Could you check a few things on this drawing? It's one solid part, dimensions in mm from its lowest x, y, z. Round coordinates to 2 decimals unless told otherwise and drop trailing zeros. Loops run counter-clockwise (first coordinate to the right, second up) from the corner with the lowest first, then second, coordinate; pieces in that order, holes last. Notation, with made-up numbers: (-29, -22) -> (-10, -22) arc R21 ccw to (-10, 15) -> close; hole circle Ø9 at (66, -9.5). An arc over 180 degrees is marked (long way). Write each question's results on one line, items separated by ' | '.
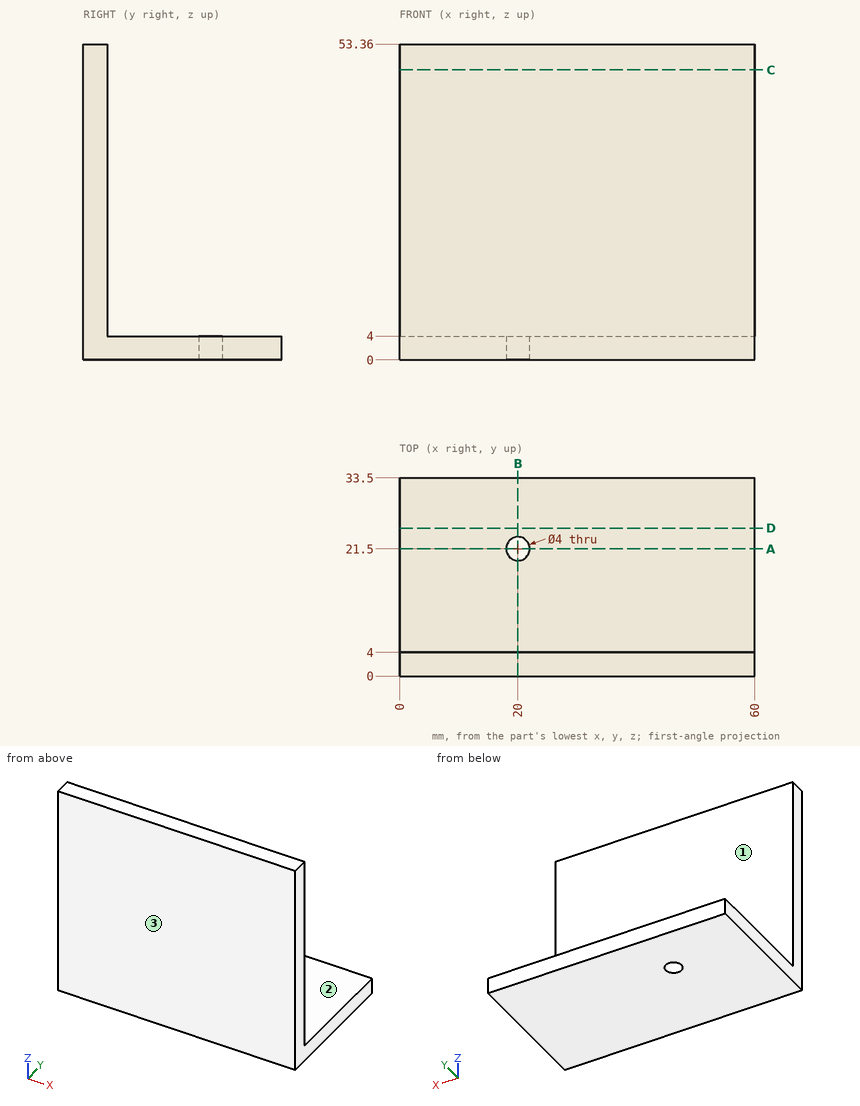
1) I need wall thicknesses on line 1 (Z direction, x = 25.5, y = 30.5); line 2 (Y direction, x = 20, z = 1). Which ranges of each line are inside material? Lowest first, please.
Model answer:
line 1: z = 0 to 4 | line 2: y = 0 to 19.5, 23.5 to 33.5
2) I want a section at B-B, the plane x = 20. Write out the boundary of the cut face in (y, z), plus the area to 3 significant figures.
Model answer:
outline: (0, 0) -> (19.5, 0) -> (19.5, 4) -> (4, 4) -> (4, 53.36) -> (0, 53.36) -> close; (23.5, 0) -> (33.5, 0) -> (33.5, 4) -> (23.5, 4) -> close | area: 315 mm2
3) I want a section at C-C, the plane z = 49. Write out the boundary of the cut face in (x, y).
Model answer:
outline: (0, 0) -> (60, 0) -> (60, 4) -> (0, 4) -> close
4) I want a section at A-A, the plane y = 21.5. Write out the boundary of the cut face in (x, z).
Model answer:
outline: (0, 0) -> (18, 0) -> (18, 4) -> (0, 4) -> close; (22, 0) -> (60, 0) -> (60, 4) -> (22, 4) -> close
5) If we mould it in two halves opening along Y, with no side actions, what happens to the marked faces 1, 2 and 3? For each: released by +Y, released by -Y, zero draft, split by the parting line, or undercut.
Model answer:
face 1: released by +Y | face 2: zero draft | face 3: released by -Y
6) I'm going to push flat-ended pins straight in: pin 1 (15 mm diameter, centred on x = 23.5, z = 36.5, fed in from +Y); pin 2 (3.5 mm diameter, centred on x = 20, y = 21.5, fed in from +Z); pin 3 (15 mm diameter, centred on x = 24.5, y = 24, fed in from +Z). Where does each tip first touch, or does it pass through?
Model answer:
pin 1: stops at y = 4 | pin 2: passes through | pin 3: stops at z = 4
